Build history of the part. All positions in model axes, mm. Face numbers are marked on the shaded views. A direction names the side the tool comes from. Coordinates: 2 decimals unless noted, no trailing zeros. Write each loop counter-clockwise with the first axis right and the second up, starting at its lowest first coordinate (ties: lowest second). Pieces come first, ordered by that corner, then holes.
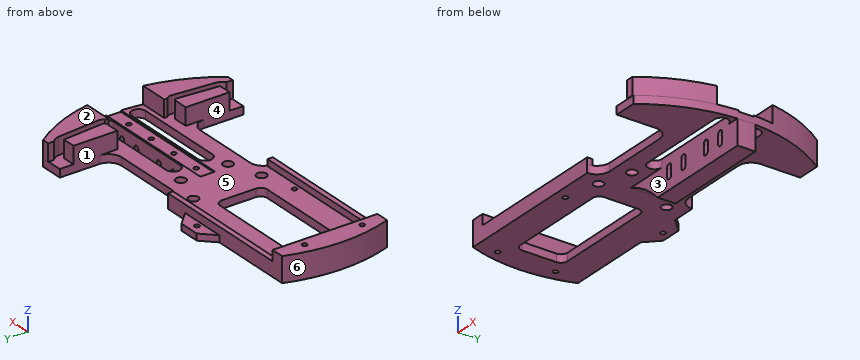
```python
from build123d import *

# Parameters (mm, degrees)
BOSS_EXTRUDE1_DEPTH     = 3.81
BOSS_EXTRUDE2_DEPTH     = 8.255
SKETCH3_W               = 63.5
SKETCH3_H               = 7.1
CUT_EXTRUDE1_DEPTH      = 0.635
CUT_EXTRUDE4_DEPTH      = 4.81
CUT_EXTRUDE5_DEPTH      = 4.81
SKETCH12_R              = 2.4257
CUT_EXTRUDE6_DEPTH      = 4.81
BOSS_EXTRUDE3_DEPTH     = 12.065
SKETCH4_R               = 1.143
CUT_EXTRUDE2_DEPTH      = 11.43
CUT_EXTRUDE7_DEPTH      = 50.016
CUT_EXTRUDE8_DEPTH      = 41.392
CUT_EXTRUDE8_DEPTH_BACK = 50.016
SKETCH17_R              = 2.413
CUT_EXTRUDE9_DEPTH      = 16.875
BOSS_EXTRUDE5_DEPTH     = 8.255
SKETCH20_W              = 69.85
SKETCH20_H              = 3.175
BOSS_EXTRUDE6_DEPTH     = 2.54
BOSS_EXTRUDE7_DEPTH     = 3.175
SKETCH22_R              = 1.18745
CUT_EXTRUDE10_DEPTH     = 13.065


with BuildPart() as part:
    # Sketch1 → Boss-Extrude1 (new body)
    with BuildSketch(Plane.XY):
        with BuildLine():
            Line((10.977415053, 19.05), (44.196, 19.05))
            ThreePointArc((44.196, 19.05), (48.686128061, 20.909871939), (50.546, 25.4))
            Line((50.546, 25.4), (50.546, 44.45))
            Line((50.546, 44.45), (61.579155694, 44.45))
            ThreePointArc((61.579155694, 44.45), (75.946, 0), (61.579155694, -44.45))
            Line((61.579155694, -44.45), (50.546, -44.45))
            Line((50.546, -44.45), (50.546, -25.4))
            ThreePointArc((50.546, -25.4), (48.686128061, -20.909871939), (44.196, -19.05))
            Line((44.196, -19.05), (10.977415053, -19.05))
            ThreePointArc((10.977415053, -19.05), (6.487286992, -20.909871939), (4.627415053, -25.4))
            Line((4.627415053, -25.4), (-71.572584947, -25.4))
            ThreePointArc((-71.572584947, -25.4), (-75.946, 0), (-71.572584947, 25.4))
            Line((-71.572584947, 25.4), (4.627415053, 25.4))
            ThreePointArc((4.627415053, 25.4), (6.487286992, 20.909871939), (10.977415053, 19.05))
        make_face()
    extrude(amount=BOSS_EXTRUDE1_DEPTH)

    # Sketch2 → Boss-Extrude2 (add)
    with BuildSketch(Plane.XY.offset(3.81)):
        with BuildLine():
            Line((61.865268471, 17.78), (60.095110466, 38.1))
            ThreePointArc((60.095110466, 38.1), (59.464196764, 40.158289632), (58.047089349, 41.778911391))
            Line((58.047089349, 41.778911391), (57.900800643, 44.704))
            Line((57.900800643, 44.704), (61.395010384, 44.704))
            ThreePointArc((61.395010384, 44.704), (69.822038137, 29.877715884), (74.728381149, 13.544887112))
            Line((74.728381149, 13.544887112), (60.759450402, 13.544887112))
            Line((60.759450402, 13.544887112), (60.759450402, 15.094127876))
            ThreePointArc((60.759450402, 15.094127876), (61.639191639, 16.302501703), (61.865268471, 17.78))
        make_face()
        with BuildLine():
            Line((58.651639318, 17.500047669), (56.881481313, 37.820047669))
            Line((56.881481313, 37.820047669), (50.546, 37.820047669))
            Line((50.546, 37.820047669), (50.546, 16.566735288))
            Line((50.546, 16.566735288), (57.366094516, 16.566735288))
            ThreePointArc((57.366094516, 16.566735288), (58.160401987, 16.824667019), (58.651639318, 17.500047669))
        make_face()
        with BuildLine():
            Line((60.759450402, -13.544887112), (74.728381149, -13.544887112))
            ThreePointArc((74.728381149, -13.544887112), (69.822038137, -29.877715884), (61.395010384, -44.704))
            Line((61.395010384, -44.704), (57.900800643, -44.704))
            Line((57.900800643, -44.704), (58.047089349, -41.778911391))
            ThreePointArc((58.047089349, -41.778911391), (59.464196764, -40.158289632), (60.095110466, -38.1))
            Line((60.095110466, -38.1), (61.865268471, -17.78))
            ThreePointArc((61.865268471, -17.78), (61.639191639, -16.302501703), (60.759450402, -15.094127876))
            Line((60.759450402, -15.094127876), (60.759450402, -13.544887112))
        make_face()
        with BuildLine():
            Line((50.546, -16.566735288), (57.366094516, -16.566735288))
            ThreePointArc((57.366094516, -16.566735288), (58.160401987, -16.824667019), (58.651639318, -17.500047669))
            Line((58.651639318, -17.500047669), (56.881481313, -37.820047669))
            Line((56.881481313, -37.820047669), (50.546, -37.820047669))
            Line((50.546, -37.820047669), (50.546, -16.566735288))
        make_face()
    extrude(amount=BOSS_EXTRUDE2_DEPTH)

    # Sketch3 → Cut-Extrude1 (cut)
    with BuildSketch(Plane.XY.offset(3.81)):
        with Locations((44.831, 0)):
            Rectangle(SKETCH3_W, SKETCH3_H)
    extrude(amount=-CUT_EXTRUDE1_DEPTH, mode=Mode.SUBTRACT)

    # Sketch9 → Cut-Extrude4 (cut, through all)
    with BuildSketch(Plane.XY.offset(3.81)):
        with BuildLine():
            Line((69.85, 11.17), (25.4, 11.17))
            ThreePointArc((25.4, 11.17), (21.971, 7.741), (25.4, 4.312))
            Line((25.4, 4.312), (69.85, 4.312))
            ThreePointArc((69.85, 4.312), (73.279, 7.741), (69.85, 11.17))
        make_face()
        with BuildLine():
            Line((69.85, -4.312), (25.4, -4.312))
            ThreePointArc((25.4, -4.312), (21.971, -7.741), (25.4, -11.17))
            Line((25.4, -11.17), (69.85, -11.17))
            ThreePointArc((69.85, -11.17), (73.279, -7.741), (69.85, -4.312))
        make_face()
    extrude(amount=-CUT_EXTRUDE4_DEPTH, mode=Mode.SUBTRACT)

    # Sketch10 → Cut-Extrude5 (cut, through all)
    with BuildSketch(Plane.XY.offset(3.81)):
        with BuildLine():
            Line((-10.922, 11.43), (-59.182, 11.43))
            ThreePointArc((-59.182, 11.43), (-61.42706403, 10.50006403), (-62.357, 8.255))
            Line((-62.357, 8.255), (-62.357, -8.255))
            ThreePointArc((-62.357, -8.255), (-61.42706403, -10.50006403), (-59.182, -11.43))
            Line((-59.182, -11.43), (-10.922, -11.43))
            ThreePointArc((-10.922, -11.43), (-8.67693597, -10.50006403), (-7.747, -8.255))
            Line((-7.747, -8.255), (-7.747, 8.255))
            ThreePointArc((-7.747, 8.255), (-8.67693597, 10.50006403), (-10.922, 11.43))
        make_face()
    extrude(amount=-CUT_EXTRUDE5_DEPTH, mode=Mode.SUBTRACT)

    # Sketch12 → Cut-Extrude6 (cut, through all)
    with BuildSketch(Plane.XY.offset(3.81)):
        with Locations((15.24, 11.43)):
            Circle(SKETCH12_R)
        with Locations((15.24, -11.43)):
            Circle(SKETCH12_R)
    extrude(amount=-CUT_EXTRUDE6_DEPTH, mode=Mode.SUBTRACT)

    # Sketch14 → Boss-Extrude3 (add)
    with BuildSketch(Plane(origin=(0, 0, 0), x_dir=(-1, 0, 0), z_dir=(0, 0, -1))):
        with BuildLine():
            Line((-75.823489579, 4.312), (7.747, 4.312))
            Line((7.747, 4.312), (7.747, -4.312))
            Line((7.747, -4.312), (-75.823489579, -4.312))
            ThreePointArc((-75.823489579, -4.312), (-75.946, 0), (-75.823489579, 4.312))
        make_face()
    extrude(amount=BOSS_EXTRUDE3_DEPTH)

    # Sketch4 → Cut-Extrude2 (cut)
    with BuildSketch(Plane.XY.offset(3.175)):
        with Locations((20.701, 0)):
            Circle(SKETCH4_R)
        with Locations((35.687, 0)):
            Circle(SKETCH4_R)
        with Locations((50.673, 0)):
            Circle(SKETCH4_R)
        with Locations((65.659, 0)):
            Circle(SKETCH4_R)
    extrude(amount=-CUT_EXTRUDE2_DEPTH, mode=Mode.SUBTRACT)

    # Sketch15 → Cut-Extrude7 (cut, through all)
    with BuildSketch(Plane(origin=(0, 4.312, 0), x_dir=(1, 0, 0), z_dir=(0, 1, 0))):
        with BuildLine():
            Line((28.8925, 1.615666853), (28.8925, 5.933666853))
            ThreePointArc((28.8925, 5.933666853), (30.2514, 7.292566853), (31.6103, 5.933666853))
            Line((31.6103, 5.933666853), (31.6103, 1.615666853))
            ThreePointArc((31.6103, 1.615666853), (30.2514, 0.256766853), (28.8925, 1.615666853))
        make_face()
        with BuildLine():
            Line((41.1099, 1.615666853), (41.1099, 5.933666853))
            ThreePointArc((41.1099, 5.933666853), (39.751, 7.292566853), (38.3921, 5.933666853))
            Line((38.3921, 5.933666853), (38.3921, 1.615666853))
            ThreePointArc((38.3921, 1.615666853), (39.751, 0.256766853), (41.1099, 1.615666853))
        make_face()
        with BuildLine():
            Line((65.5955, 1.615666853), (65.5955, 5.933666853))
            ThreePointArc((65.5955, 5.933666853), (64.2366, 7.292566853), (62.8777, 5.933666853))
            Line((62.8777, 5.933666853), (62.8777, 1.615666853))
            ThreePointArc((62.8777, 1.615666853), (64.2366, 0.256766853), (65.5955, 1.615666853))
        make_face()
        with BuildLine():
            Line((56.0959, 1.615666853), (56.0959, 5.933666853))
            ThreePointArc((56.0959, 5.933666853), (54.737, 7.292566853), (53.3781, 5.933666853))
            Line((53.3781, 5.933666853), (53.3781, 1.615666853))
            ThreePointArc((53.3781, 1.615666853), (54.737, 0.256766853), (56.0959, 1.615666853))
        make_face()
    extrude(amount=-CUT_EXTRUDE7_DEPTH, mode=Mode.SUBTRACT)

    # Sketch16 → Cut-Extrude8 (cut, two sides)
    with BuildSketch(Plane.XZ.offset(4.312)) as cut_extrude8_sk:
        with BuildLine():
            Line((4.627415053, 0), (-7.747, 0))
            Line((-7.747, 0), (-7.747, -12.065))
            Line((-7.747, -12.065), (0, -12.065))
            Line((0, -12.065), (22.547469063, -12.065))
            ThreePointArc((22.547469063, -12.065), (14.291875083, -4.986210911), (4.627415053, 0))
        make_face()
    extrude(amount=CUT_EXTRUDE8_DEPTH, mode=Mode.SUBTRACT)
    extrude(cut_extrude8_sk.sketch, amount=-CUT_EXTRUDE8_DEPTH_BACK, mode=Mode.SUBTRACT)

    # Sketch17 → Cut-Extrude9 (cut, through all)
    with BuildSketch(Plane.XY.offset(3.81)):
        with Locations((-0.127, 16.51)):
            Circle(SKETCH17_R)
        with Locations((-0.127, -16.51)):
            Circle(SKETCH17_R)
    extrude(amount=-CUT_EXTRUDE9_DEPTH, mode=Mode.SUBTRACT)

    # Sketch19 → Boss-Extrude5 (add)
    with BuildSketch(Plane.XY.offset(3.81)):
        with BuildLine():
            Line((-71.572584947, -25.4), (-65.222584947, -25.4))
            Line((-65.222584947, -25.4), (-65.222584947, 25.4))
            Line((-65.222584947, 25.4), (-71.572584947, 25.4))
            ThreePointArc((-71.572584947, 25.4), (-75.946, 0), (-71.572584947, -25.4))
        make_face()
    extrude(amount=BOSS_EXTRUDE5_DEPTH)

    # Sketch20 → Boss-Extrude6 (add)
    with BuildSketch(Plane.XZ.offset(25.4)):
        with Locations((-30.297584947, 5.3975)):
            Rectangle(SKETCH20_W, SKETCH20_H)
    boss_extrude6 = extrude(amount=-BOSS_EXTRUDE6_DEPTH)

    # Mirror1: Boss-Extrude6 across plane
    add(boss_extrude6.mirror(Plane.ZX))

    # Sketch21 → Boss-Extrude7 (add)
    with BuildSketch(Plane(origin=(0, 0, 0), x_dir=(-1, 0, 0), z_dir=(0, 0, -1))):
        Polygon((6.802584947, 25.4), (13.152584947, 31.75), (23.312584947, 31.75), (29.662584947, 25.4), align=None)
    extrude(amount=-BOSS_EXTRUDE7_DEPTH)

    # Sketch22 → Cut-Extrude10 (cut, through all)
    with BuildSketch(Plane(origin=(0, 0, 0), x_dir=(-1, 0, 0), z_dir=(0, 0, -1))):
        with Locations((18.232584947, 27.94)):
            Circle(SKETCH22_R)
        with Locations((16.962584947, -20.30328658)):
            Circle(SKETCH22_R)
        with Locations((69.032584947, 12.7)):
            Circle(SKETCH22_R)
        with Locations((69.032584947, -15.24)):
            Circle(SKETCH22_R)
    extrude(amount=-CUT_EXTRUDE10_DEPTH, mode=Mode.SUBTRACT)


solid = part.part
```
1. Saw through at B-B on x = -38.5. List the corners of the cut face in (y, z) (3 decimals).
Computed values:
outline: (-25.4, 0) - (-11.43, 0) - (-11.43, 3.81) - (-22.86, 3.81) - (-22.86, 6.985) - (-25.4, 6.985) - close; (11.43, 0) - (25.4, 0) - (25.4, 6.985) - (22.86, 6.985) - (22.86, 3.81) - (11.43, 3.81) - close
2. Probe line 1 along Z through (x, y) = (61.5, 1) (3 decimals); line 2 along X through (y, z) = (2, 4); line 3 along X through (y, z) = (-32, 9.75). List the from-to ranges inside material, lowest first.
Computed values:
line 1: z = -12.065 to 3.175
line 2: x = -75.92 to -65.22
line 3: x = 50.55 to 57.39, 60.63 to 68.88
3. Saw through at C-C on x = 15.24. List the corners of the cut face in (y, z) (3 decimals).
Computed values:
outline: (-19.05, 0) - (-13.856, 0) - (-13.856, 3.81) - (-19.05, 3.81) - close; (-9.004, 0) - (-4.312, 0) - (-4.312, -5.642) - (4.312, -5.642) - (4.312, 0) - (9.004, 0) - (9.004, 3.81) - (3.55, 3.81) - (3.55, 3.175) - (-3.55, 3.175) - (-3.55, 3.81) - (-9.004, 3.81) - close; (13.856, 0) - (19.05, 0) - (19.05, 3.81) - (13.856, 3.81) - close
4. Saw through at A-A on z = -3.5. List the corners of the cut face in (x, y), plus the area to 3 significant figures.
Computed values:
outline: (11.94, -4.31) - (28.89, -4.31) - (28.89, 4.31) - (11.94, 4.31) - close; (31.61, -4.31) - (38.39, -4.31) - (38.39, 4.31) - (31.61, 4.31) - close; (41.11, -4.31) - (53.38, -4.31) - (53.38, 4.31) - (41.11, 4.31) - close; (56.1, -4.31) - (62.88, -4.31) - (62.88, 4.31) - (56.1, 4.31) - close; (65.6, -4.31) - (75.82, -4.31) arc R75.95 ccw to (75.82, 4.31) - (65.6, 4.31) - (65.6, 1.14) arc R1.14 cw (long way) to (65.6, -1.14) - close; hole circle Ø2.29 at (20.7, 0); hole circle Ø2.29 at (35.69, 0); hole circle Ø2.29 at (50.67, 0)
area: 443 mm2
5. Saw through at D-D on y = 34. List the corners of the cut face in (x, z) (3 decimals), plus the area to 3 significant figures.
Computed values:
outline: (50.546, 0) - (67.91, 0) - (67.91, 12.065) - (60.452, 12.065) - (60.452, 3.81) - (57.214, 3.81) - (57.214, 12.065) - (50.546, 12.065) - close
area: 183 mm2
6. 3-axis set-ups, long thin cutter, end or side, ignore diameter. For the marked faces 1, 2 and 3: which of +Z, -Z, +X, -X, +Y, -Y reach the whole face in a straight line?
Computed values:
face 1: +Z, +Y
face 2: +Z, +X, -X, +Y, -Y
face 3: -Z
7. Flat gauge pins, fed straight in: pin 1 (1.3 mm diameter, centred on y = -1.5, z = -4, fed in from +X); pin 2 (12 mm diameter, centred on x = 18.5, y = -9.5, fed in from +Z); pin 3 (2 mm diameter, centred on x = -18.23, y = 27.94, fed in from +Z); pin 4 (1.1 mm diameter, centred on x = 20.5, y = 0.5, fed in from +Z) (3 decimals). Where does each tip first touch, or does it go through?
Computed values:
pin 1: stops at x = 75.94
pin 2: stops at z = 3.81
pin 3: passes through
pin 4: stops at z = -8.255
8. Mould opens along Y. For the marked faces 4, 5 and 6 say: +Y half, -Y half, draft (parallel to the pull), parting line (faces both ways), or undercut.
Computed values:
face 4: draft
face 5: undercut
face 6: parting line
